Autodesk Inventor part; units mm, degrees
ref_plane "Work Plane1" through (0, 0, -2.5) normal (0, 0, 1) x (1, 0, 0)
ref_plane "YZ Plane" through (0, 0, 0) normal (1, 0, 0) x (0, 1, 0)
ref_plane "XZ Plane" through (0, 0, 0) normal (0, 1, 0) x (-1, 0, 0)
ref_plane "Work Plane1" through (0, 0, -2.5) normal (0, 0, 1) x (1, 0, 0)
sketch "Sketch1" plane through (0, 0, -2.5) normal (0, 0, 1) x (1, 0, 0)
  circle A0 centre (0, 0) radius 2.34
extrude "Extrusion3" add sketch "Sketch1" along normal blind 2.5
sketch "Sketch2" plane through (0, 0, 0) normal (0, 0, 1) x (1, 0, 0)
  circle A0 centre (0, 0) radius 1.25
extrude "Extrusion2" add sketch "Sketch2" along normal blind 6
sketch "Sketch3" plane through (0, 0, -2.5) normal (0, 0, 1) x (1, 0, 0)
  line L0 (0.5947, -1.03) -> (-0.5947, -1.03)
  line L1 (0.5947, 1.03) -> (1.1893, 0)
  line L2 (-0.5947, -1.03) -> (-1.1893, 0)
  line L3 (-1.1893, 0) -> (-0.5947, 1.03)
  line L4 (1.1893, 0) -> (0.5947, -1.03)
  line L5 (-0.5947, 1.03) -> (0.5947, 1.03)
extrude "Extrusion1" cut sketch "Sketch3" along normal blind 2.5
fillet "Fillet1" radius 0.1 2 edges at (-2.34, 0, 0) (-2.34, 0, -2.5)
chamfer "Chamfer1" distance 0.2 angle 45 1 edges at (-1.25, 0, 6)
properties part number "M2.5 x 6mm SHCS"
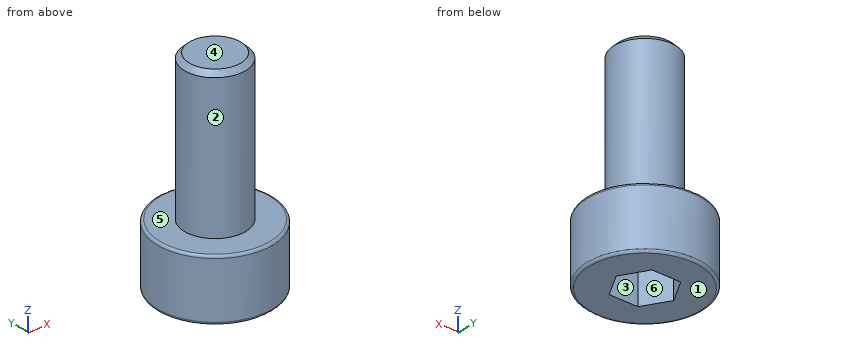
For this review, take the finished solid that the model builds, in its own axes (mm). Face numbers are marked on the shaded views. A direction names the side the tool comes from. Round coordinates to 2 decimals unless told otherwise and drop trailing zeros. Loops run counter-clockwise (first coordinate to the right, second up) from the corner with the lowest first, then second, coordinate; pieces in that order, holes last.
Q1. Add section B-B on x = 0. Write out the cut boundary in (y, z).
Result sheet:
outline: (-2.34, -2.4) arc R0.1 ccw to (-2.24, -2.5) - (-1.03, -2.5) - (-1.03, 0) - (1.03, 0) - (1.03, -2.5) - (2.24, -2.5) arc R0.1 ccw to (2.34, -2.4) - (2.34, -0.1) arc R0.1 ccw to (2.24, 0) - (1.25, 0) - (1.25, 5.8) - (1.05, 6) - (-1.05, 6) - (-1.25, 5.8) - (-1.25, 0) - (-2.24, 0) arc R0.1 ccw to (-2.34, -0.1) - close
Q2. Machinability: for the marked faces 4, 5 and 6, which of the approach directions +Z, -Z, +X, -X, +Y, -Y give a long, thin tool a straight path to every point of the face, cutting with its end or side? Answer none if there is none.
Result sheet:
face 4: +Z, +X, -X, +Y, -Y
face 5: +Z
face 6: -Z
Q3. To check wall thickness, follow line 1 along Y through (x, z) = (1.1, 2); line 2 along Z through (x, y) = (-2.1, 0.35); line 3 along Y through (x, z) = (-0.55, -0.5). State the ranges of each line that lie inside material, in increasing order.
Result sheet:
line 1: y = -0.59 to 0.59
line 2: z = -2.5 to 0
line 3: y = -2.27 to -1.03, 1.03 to 2.27
Q4. Insertion check: pin 1 Ø1 at (x, z) = (1.5, -0.5) entering from -Y. The pin has a flat end and moves straight along its axis. Give the tip position at first contact, or say it passes through.
Result sheet:
pin 1: stops at y = -2.12
Q5. Add section C-C on z = 4.5. Write out the cut boundary in (x, y), plus the area to 3 significant figures.
Result sheet:
outline: circle Ø2.5 at (0, 0)
area: 4.91 mm2
Q6. Add section A-A on z = -0.5. Write out the cut boundary in (x, y), plus the area to 3 significant figures.
Result sheet:
outline: circle Ø4.68 at (0, 0); hole (-1.19, 0) - (-0.59, -1.03) - (0.59, -1.03) - (1.19, 0) - (0.59, 1.03) - (-0.59, 1.03) - close
area: 13.5 mm2
Q7. Mouldability with a two-part tool opening along X and no side actions: class the marked faces 1, 2 and 3 as +X half, -X half, draft (parallel to the pull), parting line (faces both ways), or undercut.
Result sheet:
face 1: draft
face 2: parting line
face 3: undercut
